Autodesk Inventor part; units mm, degrees
ref_plane "YZ Plane" through (0, 0, 0) normal (1, 0, 0) x (0, 1, 0)
ref_plane "XZ Plane" through (0, 0, 0) normal (0, 1, 0) x (-1, 0, 0)
ref_plane "XY Plane" through (0, 0, 0) normal (0, 0, 1) x (1, 0, 0)
sketch "Skizze1" plane through (0, 0, 0) normal (1, 0, 0) x (0, 1, 0)
  line L0 (0, 0) -> (40, 0)
  line L1 (40, 0) -> (40, -50)
  line L2 (40, -50) -> (0, -50)
  line L3 (0, -50) -> (0, 0)
  dimension "d0" = 40
  dimension "d1" = 50
extrude "Extrusion1" add sketch "Skizze1" along normal blind 40
sketch "Skizze2" plane through (0, 0, 0) normal (0, 0, 1) x (1, 0, 0)
  line L0 (0, 40) -> (40, 40) construction
  line L1 (0, 0) -> (40, 40) construction
  line L2 (0, 40) -> (40, 0) construction
  line L3 (40, 40) -> (40, 0) construction
  circle A0 centre (20, 20) radius 12.5
  dimension "d4" = 25
extrude "Extrusion2" add sketch "Skizze2" along normal blind 20
sketch "Skizze3" plane through (40, 0, 0) normal (1, 0, 0) x (0, 0, -1)
  line L0 (3.2137, 16.0634) -> (29.2155, 16.0634) construction
  line L1 (29.2155, 16.0634) -> (29.2155, 5.0626) construction
  line L2 (29.2155, 5.0626) -> (3.2137, 5.0626) construction
  line L3 (3.2137, 5.0626) -> (3.2137, 16.0634) construction
  point P0 (0, 0)
properties part number "kamera_dummy"
The model under review builds one solid part; all positions refer to its coordinate system, in mm. A direction names the side the tool comes from. Round coordinates to 2 decimals unless told otherwise and drop trailing zeros. Write each loop counter-clockwise with the first axis right and the second up, starting at its lowest first coordinate (ties: lowest second). Pieces come first, ordered by that corner, then holes.
(1) Insertion check: pin 1 (10 mm diameter, centred on x = 15.5, z = 8.5, fed in from -Y); pin 2 (12 mm diameter, centred on x = 27, z = 7, fed in from +Y); pin 3 (3 mm diameter, centred on x = 29, z = 11, fed in from +Y). Each pin has a flat end and moves straight along its axis. Give the tip position at first contact, or say it passes through.
(2) We need section A-A on y = 20. Give the boundary of the cut face in (x, z).
(3) Machinability: for faces 5 (the flat face through (20, 20, -50)), 6 (the flat face through (11, 11, 0)), which of the approach directions +Z, -Z, +X, -X, +Y, -Y give a long, thin tool a straight path to every point of the face, cutting with its end or side? Answer none if there is none.
(4) We need section C-C on x = 6. Give the boundary of the cut face in (y, z).
(5) Mouldability with a two-part tool opening along Y and no side actions: class faces 1 (the flat face through (20, 0, -25)), 2 (the flat face through (40, 20, -25)), 3 (the cylindrical face through (31.547, 24.788, 9.86)), 4 (the flat face through (20, 40, -25)) as +Y half, -Y half, draft (parallel to the pull), parting line (faces both ways), or undercut.
(6) Wall thickness on L1, parallel to Z at x = 15, y = 8; L2, parallel to X at y = 24.5, z = 2; L3, parallel to Y at x = 18, z = 14: over which ranges is each line inside the solid? List them lowest first.
Findings below:
1. pin 1: stops at y = 7.5
1. pin 2: stops at y = 32.46
1. pin 3: stops at y = 30
2. outline: (0, -50) - (40, -50) - (40, 0) - (32.5, 0) - (32.5, 20) - (7.5, 20) - (7.5, 0) - (0, 0) - close
3. face 5: -Z, +X, -X, +Y, -Y
3. face 6: +Z
4. outline: (0, -50) - (40, -50) - (40, 0) - (0, 0) - close
5. face 1: -Y half
5. face 2: draft
5. face 3: parting line
5. face 4: +Y half
6. L1: z = -50 to 0
6. L2: x = 8.34 to 31.66
6. L3: y = 7.66 to 32.34
